The model under review builds one solid part; all positions refer to its coordinate system, in mm. A direction names the side the tool comes from. Coordinates: 2 decimals unless noted, no trailing zeros. Loops run counter-clockwise (first coordinate to the right, second up) from the corner with the lowest first, then second, coordinate; pieces in that order, holes last. Notation, with made-up numbers: M -39,54.25 L -4,54.25 A13 ccw -4,58.25 Z; hole C -26,55 d3. An arc over 180 degrees is marked long. Use one line per item in the form item = value.
```python
from build123d import *

# Parameters (mm, degrees)
EXTRUDE_1_DEPTH     = 9
SKETCH_2_W          = 12
SKETCH_2_H          = 9
EXTRUDE_2_DEPTH     = 6
EXTRUDE_3_DEPTH     = 23
EXTRUDE_4_DEPTH     = 8
SKETCH_6_R          = 1.5
CUT_EXTRUDE_1_DEPTH = 8
SKETCH_6_3_R        = 11
EXTRUDE_5_DEPTH     = 2
SKETCH_7_R          = 2.5
EXTRUDE_6_DEPTH     = 21


with BuildPart() as part:
    # Sketch 1 → Extrude 1 (new body)
    with BuildSketch(Plane(origin=(0, 0, 0), x_dir=(1, 0, 0), z_dir=(0, 1, 0))):
        with BuildLine():
            ThreePointArc((-13.564659966, 21), (-15.709241166, 19.447872428), (-17.67766953, 17.67766953))
            Line((-17.67766953, 17.67766953), (0, 0))
            Line((0, 0), (17.67766953, 17.67766953))
            ThreePointArc((17.67766953, 17.67766953), (15.709241166, 19.447872428), (13.564659966, 21))
            Line((13.564659966, 21), (-13.564659966, 21))
        make_face()
        with BuildLine():
            Line((0, 0), (-17.67766953, 17.67766953))
            ThreePointArc((-17.67766953, 17.67766953), (-19.447872428, 15.709241166), (-21, 13.564659966))
            Line((-21, 13.564659966), (-21, -13.564659966))
            ThreePointArc((-21, -13.564659966), (-19.447872428, -15.709241166), (-17.67766953, -17.67766953))
            Line((-17.67766953, -17.67766953), (0, 0))
        make_face()
        with BuildLine():
            Line((17.67766953, -17.67766953), (0, 0))
            Line((0, 0), (-17.67766953, -17.67766953))
            ThreePointArc((-17.67766953, -17.67766953), (-15.709241166, -19.447872428), (-13.564659966, -21))
            Line((-13.564659966, -21), (13.564659966, -21))
            ThreePointArc((13.564659966, -21), (15.709241166, -19.447872428), (17.67766953, -17.67766953))
        make_face()
        with BuildLine():
            Line((17.67766953, 17.67766953), (0, 0))
            Line((0, 0), (17.67766953, -17.67766953))
            ThreePointArc((17.67766953, -17.67766953), (19.447872428, -15.709241166), (21, -13.564659966))
            Line((21, -13.564659966), (21, 13.564659966))
            ThreePointArc((21, 13.564659966), (19.447872428, 15.709241166), (17.67766953, 17.67766953))
        make_face()
    extrude(amount=EXTRUDE_1_DEPTH)

    # Sketch 2 → Extrude 2 (add)
    with BuildSketch(Plane.XY.offset(21)):
        with Locations((0, 4.5)):
            Rectangle(SKETCH_2_W, SKETCH_2_H)
    extrude(amount=EXTRUDE_2_DEPTH)

    # Sketch 4 → Extrude 3 (add)
    with BuildSketch(Plane(origin=(0, 9, 0), x_dir=(1, 0, 0), z_dir=(0, 1, 0))):
        with BuildLine():
            Line((-20.9, -13.535139453), (-20.9, 13.535139453))
            ThreePointArc((-20.9, 13.535139453), (-17.606958852, 17.606958852), (-13.535139453, 20.9))
            Line((-13.535139453, 20.9), (13.535139453, 20.9))
            ThreePointArc((13.535139453, 20.9), (17.606958852, 17.606958852), (20.9, 13.535139453))
            Line((20.9, 13.535139453), (20.9, -13.535139453))
            ThreePointArc((20.9, -13.535139453), (17.606958852, -17.606958852), (13.535139453, -20.9))
            Line((13.535139453, -20.9), (-13.535139453, -20.9))
            ThreePointArc((-13.535139453, -20.9), (-17.606958852, -17.606958852), (-20.9, -13.535139453))
        make_face()
    extrude(amount=EXTRUDE_3_DEPTH)

    # Sketch 5 → Extrude 4 (add)
    with BuildSketch(Plane(origin=(0, 32, 0), x_dir=(1, 0, 0), z_dir=(0, 1, 0))):
        with BuildLine():
            Line((21, -13.564659966), (21, 13.564659966))
            ThreePointArc((21, 13.564659966), (17.67766953, 17.67766953), (13.564659966, 21))
            Line((13.564659966, 21), (-13.564659966, 21))
            ThreePointArc((-13.564659966, 21), (-17.67766953, 17.67766953), (-21, 13.564659966))
            Line((-21, 13.564659966), (-21, -13.564659966))
            ThreePointArc((-21, -13.564659966), (-17.67766953, -17.67766953), (-13.564659966, -21))
            Line((-13.564659966, -21), (13.564659966, -21))
            ThreePointArc((13.564659966, -21), (17.67766953, -17.67766953), (21, -13.564659966))
        make_face()
    extrude(amount=EXTRUDE_4_DEPTH)

    # Sketch 6 → Cut-Extrude 1 (cut)
    with BuildSketch(Plane(origin=(0, 40, 0), x_dir=(1, 0, 0), z_dir=(0, 1, 0))):
        with Locations(Location((-15.5, -15.5, 0), (0, 0, 270))):
            Circle(SKETCH_6_R)
        with Locations(Location((-15.5, 15.5, 0), (0, 0, 270))):
            Circle(SKETCH_6_R)
        with Locations(Location((15.5, 15.5, 0), (0, 0, 270))):
            Circle(SKETCH_6_R)
        with Locations(Location((15.5, -15.5, 0), (0, 0, 270))):
            Circle(SKETCH_6_R)
    extrude(amount=-CUT_EXTRUDE_1_DEPTH, mode=Mode.SUBTRACT)

    # Sketch 6_3 → Extrude 5 (add)
    with BuildSketch(Plane(origin=(0, 40, 0), x_dir=(1, 0, 0), z_dir=(0, 1, 0))):
        with Locations(Location((0, 0, 0), (0, 0, 270))):
            Circle(SKETCH_6_3_R)
    extrude(amount=EXTRUDE_5_DEPTH)

    # Sketch 7 → Extrude 6 (add)
    with BuildSketch(Plane(origin=(0, 42, 0), x_dir=(1, 0, 0), z_dir=(0, 1, 0))):
        with Locations(Location((0, 0, 0), (0, 0, 90))):
            Circle(SKETCH_7_R)
    extrude(amount=EXTRUDE_6_DEPTH)


solid = part.part
```
1. Wall thickness on line 1 along X through (y, z) = (36.75, -15.5); line 2 along Z through (x, y) = (-15, 37); line 3 along Z through (x, y) = (4, 35): over which ranges is each line inside the solid? List them lowest first. Write a range as from..to.
Response values:
line_1 = -19.62..-17, -14..14, 17..19.62
line_2 = -20..-16.91, -14.09..14.09, 16.91..20
line_3 = -21..21
2. Add section A-A (y = 36). State the section outline as (x, z) points.
Response values:
outline = M -21,-13.56 A25 ccw -13.56,-21 L 13.56,-21 A25 ccw 21,-13.56 L 21,13.56 A25 ccw 13.56,21 L -13.56,21 A25 ccw -21,13.56 Z; hole C -15.5,-15.5 d3; hole C -15.5,15.5 d3; hole C 15.5,-15.5 d3; hole C 15.5,15.5 d3
3. Add section C-C (z = 0). State the section outline as (x, y) points.
Response values:
outline = M -21,0 L 21,0 L 21,9 L 20.9,9 L 20.9,32 L 21,32 L 21,40 L 11,40 L 11,42 L 2.5,42 L 2.5,63 L -2.5,63 L -2.5,42 L -11,42 L -11,40 L -21,40 L -21,32 L -20.9,32 L -20.9,9 L -21,9 Z
4. Insertion check: P1, Ø7, axis at y = 20, z = 3, coming from the +X side; P2, Ø0.9, axis at x = 15, z = 16, coming from the +Y side; P3, Ø2.5, axis at x = -15, z = 15.5, coming from the +Y side. Each pin has a flat end and moves straight along its axis. Give the tip position at first contact, or say it passes through.
Response values:
P1 = 20.9
P2 = 32
P3 = 40
5. Add section B-B (x = 0). State the section outline as (y, z) points.
Response values:
outline = M 0,-21 L 9,-21 L 9,-20.9 L 32,-20.9 L 32,-21 L 40,-21 L 40,-11 L 42,-11 L 42,-2.5 L 63,-2.5 L 63,2.5 L 42,2.5 L 42,11 L 40,11 L 40,21 L 32,21 L 32,20.9 L 9,20.9 L 9,27 L 0,27 Z
6. The part is to be moulded in two halves that separate along Y. For faces 1 (the face through (-15, 32, 15)), 2 (the face through (0, 20, 20.9)), 3 (the face through (15.57, 36.06, -17)), say which applies: pulls with the +Y half, pulls with the -Y half, needs draft (parallel to the pull), parting line crosses it, or undercut.
Response values:
face_1 = pulls with the +Y half
face_2 = undercut
face_3 = needs draft
7. Machinability: for faces 4 (the face through (0, 20, -20.9)), 5 (the face through (-20.9, 20, 0)), 6 (the face through (15.57, 36.06, 14)), which of the approach directions +Z, -Z, +X, -X, +Y, -Y give a long, thin tool a straight path to every point of the face, cutting with its end or side? Answer none if there is none.
Response values:
face_4 = -Z, +X, -X
face_5 = +Z, -Z, -X
face_6 = +Y
8. Add section D-D (y = 47). State the section outline as (x, z) points, then the cut area to 3 significant figures.
Response values:
outline = C 0,0 d5
area = 19.6 mm^2
